from build123d import *

# Parameters (mm, degrees)
F0_W     = 88.9
F0_H     = 63.5
F1_DEPTH = 63.5
F3_DEPTH = 63.501
F4_W     = 38.1
F4_H     = 26.7130212291
F5_DEPTH = 25.4
F6_W     = 25.4
F6_H     = 38.1
F7_DEPTH = 40.132
F9_DEPTH = 27.94


with BuildPart() as f1:
    # F0 (on Top) → F1 (new body)
    with BuildSketch(Plane.XY):
        with Locations((-1.7257053405, -12.9154672953)):
            Rectangle(F0_W, F0_H)
    extrude(amount=F1_DEPTH)

    # F2 (on face) → F3 (cut, through all)
    with BuildSketch(Plane.XZ.offset(44.6654672953)):
        Polygon((42.7242946595, 63.5), (-8.1487037241, 63.5), (42.7242946595, 0), align=None)
    extrude(amount=-F3_DEPTH, mode=Mode.SUBTRACT)

    # F4 (on face) → F5 (join)
    with BuildSketch(Plane(origin=(26.0221932234, 0, 20.8476691936), x_dir=(0, 1, 0), z_dir=(0.7804309746, 0, 0.6252419482))):
        with Locations((-0.2154672953, -13.3565106146)):
            Rectangle(F4_W, F4_H)
    extrude(amount=F5_DEPTH)

    # F6 (on face) → F7 (cut)
    with BuildSketch(Plane(origin=(0, 0, 0), x_dir=(0.7804309746, 0, 0.6252419482), z_dir=(-0.6252419482, 0, 0.7804309746))):
        with Locations((46.0433629222, -0.2154672953)):
            Rectangle(F6_W, F6_H)
    extrude(amount=-F7_DEPTH, mode=Mode.SUBTRACT)

    # F8 (on face) → F9 (join)
    with BuildSketch(Plane(origin=(0, 18.8345327047, 0), x_dir=(-1, 0, 0), z_dir=(0, 1, 0))):
        Polygon((-42.7242946595, 0), (-22.9904382266, 24.6319250545), (-42.7242946595, 24.6319250545), align=None)
    extrude(amount=-F9_DEPTH)


solid = f1.part
For this review, take the finished solid that the model builds, in its own axes (mm). A direction names the side the tool comes from. Coordinates: 2 decimals unless noted, no trailing zeros. Loops run counter-clockwise (first coordinate to the right, second up) from the corner with the lowest first, then second, coordinate; pieces in that order, holes last. Notation, with made-up numbers: (61.25, 10) -> (100.25, 10) arc R17 ccw to (100.25, 19) -> close; hole circle Ø1 at (-20.75, 57). An arc over 180 degrees is marked (long way). Write each question's results on one line, items separated by ' | '.
Q1. Add section C-C, the plane z = 15.5. State the section outline as (x, y) points, then the cut area to 3 significant figures.
Taken from the geometry:
outline: (-46.18, -44.67) -> (30.31, -44.67) -> (30.31, -9.11) -> (42.72, -9.11) -> (42.72, 18.83) -> (-46.18, 18.83) -> close | area: 5,200 mm²
Q2. For pin 1 Ø21.5 at (x, y) = (31, 9) entering from +Z, flat-tipped, find the tip position at first contact; note if it passes through.
Taken from the geometry:
pin 1: z = 28.05
Q3. Add section D-D, the plane y = -29.5. State the section outline as (x, z) points.
Taken from the geometry:
outline: (-46.18, 0) -> (42.72, 0) -> (-8.15, 63.5) -> (-46.18, 63.5) -> close
Q4. To check wall thickness, follow line 1 along Z through (x, y) = (-2, -11.5); line 2 along Z through (x, y) = (13.5, -29.5); line 3 along X through (y, z) = (-32.5, 24.5). State the ranges of each line that lie inside material, in increasing order. Write a range as [from, to].
Taken from the geometry:
line 1: [0, 55.83] | line 2: [0, 36.48] | line 3: [-46.18, 23.1]
Q5. Add section A-A, the plane y = -5. State the section outline as (x, z) points, then the cut area to 3 significant figures.
Taken from the geometry:
outline: (-46.18, 0) -> (42.72, 0) -> (42.72, 24.63) -> (22.99, 24.63) -> (-8.15, 63.5) -> (-46.18, 63.5) -> close | area: 4,270 mm²
Q6. Add section B-B, the plane x = 30. State the section outline as (y, z) points, then the cut area to 3 significant figures.
Taken from the geometry:
outline: (-44.67, 0) -> (18.83, 0) -> (18.83, 24.63) -> (-9.11, 24.63) -> (-9.11, 15.88) -> (-44.67, 15.88) -> close | area: 1,250 mm²
Q7. Machinability: for faces 1 (the flat face through (35, -9.105, 15)), 2 (the flat face through (33, 5, 24.632)), 3 (the flat face through (42.724, 5, 12)), which of the approach directions +Z, -Z, +X, -X, +Y, -Y give a long, thin tool a straight path to every point of the face, cutting with its end or side? Answer none if there is none.
Taken from the geometry:
face 1: +Z, +X, -Y | face 2: +Z, +X, +Y, -Y | face 3: +Z, -Z, +X, +Y, -Y
